from build123d import *

# Parameters (mm, degrees)
BOSS_EXTRUDE2_DEPTH = 87
CUT_EXTRUDE1_DEPTH  = 29.5
SKETCH3_R           = 1
CUT_EXTRUDE2_DEPTH  = 130.771336418
SKETCH4_R           = 1.7
CUT_EXTRUDE3_DEPTH  = 10
BOSS_EXTRUDE3_START = 2
BOSS_EXTRUDE3_DEPTH = 2
BOSS_EXTRUDE4_START = 6
BOSS_EXTRUDE4_DEPTH = 6
SKETCH7_W           = 73
SKETCH7_H           = 5.446782016
SKETCH7_H_2         = 6
CUT_EXTRUDE4_DEPTH  = 7
SKETCH8_R           = 1
CUT_EXTRUDE5_DEPTH  = 136.438914135
SKETCH9_R           = 2.5
CUT_EXTRUDE6_DEPTH  = 32
SKETCH11_W          = 10.498637593
SKETCH11_H          = 26.999999931
BOSS_EXTRUDE6_DEPTH = 23
SKETCH12_W          = 73
SKETCH12_H          = 6
SKETCH12_H_2        = 5.446782016
BOSS_EXTRUDE7_DEPTH = 14


with BuildPart() as part:
    # Sketch1 → Boss-Extrude2 (new body)
    with BuildSketch(Plane(origin=(89.94373008, 0, 0), x_dir=(0, 0, -1), z_dir=(1, 0, 0))):
        with BuildLine():
            Line((-104.016306216, 83.836001664), (-104.016306216, 0.836001664))
            ThreePointArc((-104.016306216, 0.836001664), (-62.516306216, 42.336001664), (-104.016306216, 83.836001664))
        make_face()
    extrude(amount=-BOSS_EXTRUDE2_DEPTH)

    # Sketch2 → Cut-Extrude1 (cut)
    with BuildSketch(Plane.XY.offset(104.016306216)):
        with BuildLine():
            Line((89.94373008, 55.836001595), (79.445092487, 55.836001664))
            Line((79.445092487, 55.836001664), (40.551337791, 64.805487997))
            ThreePointArc((40.551337791, 64.805487997), (5.067466824, 42.109927869), (40.551337791, 19.414367741))
            Line((40.551337791, 19.414367741), (79.445092487, 28.836001664))
            Line((79.445092487, 28.836001664), (89.94373008, 28.836001664))
            Line((89.94373008, 28.836001664), (89.94373008, 55.836001595))
        make_face()
    extrude(amount=-CUT_EXTRUDE1_DEPTH, mode=Mode.SUBTRACT)

    # Sketch3 → Cut-Extrude2 (cut, through all)
    with BuildSketch(Plane(origin=(0, 0, 62.516306216), x_dir=(-1, 0, 0), z_dir=(0, 0, -1))):
        with Locations(Location((-42.657418818, 50.264258545, 0), (0, 0, 90))):
            Circle(SKETCH3_R)
        with Locations(Location((-21.913136148, 54.699879864, 0), (0, 0, 90))):
            Circle(SKETCH3_R)
        with Locations(Location((-38.2217975, 29.519975875, 0), (0, 0, 90))):
            Circle(SKETCH3_R)
        with Locations(Location((-17.477514829, 33.955597193, 0), (0, 0, 90))):
            Circle(SKETCH3_R)
    extrude(amount=-CUT_EXTRUDE2_DEPTH, mode=Mode.SUBTRACT)

    # Sketch4 → Cut-Extrude3 (cut)
    with BuildSketch(Plane(origin=(0, 0, 62.516306216), x_dir=(-1, 0, 0), z_dir=(0, 0, -1))):
        with Locations(Location((-42.657418818, 50.264258545, 0), (0, 0, 90))):
            Circle(SKETCH4_R)
        with Locations(Location((-21.913136148, 54.699879864, 0), (0, 0, 90))):
            Circle(SKETCH4_R)
        with Locations(Location((-38.2217975, 29.519975875, 0), (0, 0, 90))):
            Circle(SKETCH4_R)
        with Locations(Location((-17.477514829, 33.955597193, 0), (0, 0, 90))):
            Circle(SKETCH4_R)
    extrude(amount=-CUT_EXTRUDE3_DEPTH, mode=Mode.SUBTRACT)

    # Sketch5 → Boss-Extrude3 (add)
    with BuildSketch(Plane(origin=(89.94373008, 0, 0), x_dir=(0, 0, -1), z_dir=(1, 0, 0)).offset(BOSS_EXTRUDE3_START)):
        with BuildLine():
            Line((-104.016306216, 55.836001595), (-104.016306216, 47.336001664))
            ThreePointArc((-104.016306216, 47.336001664), (-99.016306216, 42.336001664), (-104.016306216, 37.336001664))
            Line((-104.016306216, 37.336001664), (-104.016306216, 28.836001664))
            Line((-104.016306216, 28.836001664), (-104.016306216, 0.836001664))
            ThreePointArc((-104.016306216, 0.836001664), (-62.516306216, 42.336001664), (-104.016306216, 83.836001664))
            Line((-104.016306216, 83.836001664), (-104.016306216, 55.836001595))
        make_face()
    extrude(amount=-BOSS_EXTRUDE3_DEPTH)

    # Sketch6 → Boss-Extrude4 (add)
    with BuildSketch(Plane(origin=(91.94373008, 0, 0), x_dir=(0, 0, -1), z_dir=(1, 0, 0)).offset(BOSS_EXTRUDE4_START)):
        with BuildLine():
            Line((-104.016306216, 56.336001664), (-104.016306216, 47.336001664))
            ThreePointArc((-104.016306216, 47.336001664), (-99.016306216, 42.336001664), (-104.016306216, 37.336001664))
            Line((-104.016306216, 37.336001664), (-104.016306216, 28.336001664))
            ThreePointArc((-104.016306216, 28.336001664), (-90.016306216, 42.336001664), (-104.016306216, 56.336001664))
        make_face()
    extrude(amount=-BOSS_EXTRUDE4_DEPTH)

    # Sketch7 → Cut-Extrude4 (cut)
    with BuildSketch(Plane.XY.offset(104.016306216)):
        with Locations((47.44373008, 76.112610656)):
            Rectangle(SKETCH7_W, SKETCH7_H)
        with Locations((47.44373008, 8.836001664)):
            Rectangle(SKETCH7_W, SKETCH7_H_2)
    extrude(amount=-CUT_EXTRUDE4_DEPTH, mode=Mode.SUBTRACT)

    # Sketch8 → Cut-Extrude5 (cut, through all)
    with BuildSketch(Plane(origin=(0, 0, 62.516306216), x_dir=(-1, 0, 0), z_dir=(0, 0, -1))):
        with Locations(Location((-84.94373008, 65.836001664, 0), (0, 0, 90))):
            Circle(SKETCH8_R)
        with Locations(Location((-84.94373008, 17.836001664, 0), (0, 0, 90))):
            Circle(SKETCH8_R)
        with Locations(Location((-9.94373008, 65.836001664, 0), (0, 0, 90))):
            Circle(SKETCH8_R)
        with Locations(Location((-9.94373008, 17.836001664, 0), (0, 0, 90))):
            Circle(SKETCH8_R)
    extrude(amount=-CUT_EXTRUDE5_DEPTH, mode=Mode.SUBTRACT)

    # Sketch9 → Cut-Extrude6 (cut)
    with BuildSketch(Plane(origin=(0, 0, 62.516306216), x_dir=(-1, 0, 0), z_dir=(0, 0, -1))):
        with Locations(Location((-84.94373008, 65.836001664, 0), (0, 0, 90))):
            Circle(SKETCH9_R)
        with Locations(Location((-84.94373008, 17.836001664, 0), (0, 0, 90))):
            Circle(SKETCH9_R)
        with Locations(Location((-9.94373008, 65.836001664, 0), (0, 0, 90))):
            Circle(SKETCH9_R)
        with Locations(Location((-9.94373008, 17.836001664, 0), (0, 0, 90))):
            Circle(SKETCH9_R)
    extrude(amount=-CUT_EXTRUDE6_DEPTH, mode=Mode.SUBTRACT)

    # Sketch11 → Boss-Extrude6 (add)
    with BuildSketch(Plane.XY.offset(74.516306216)):
        with Locations((84.694411284, 42.33600163)):
            Rectangle(SKETCH11_W, SKETCH11_H)
    extrude(amount=BOSS_EXTRUDE6_DEPTH)

    # Sketch12 → Boss-Extrude7 (add)
    with BuildSketch(Plane(origin=(0, 0, 97.016306216), x_dir=(-1, 0, 0), z_dir=(0, 0, -1))):
        with Locations((-47.44373008, 8.836001664)):
            Rectangle(SKETCH12_W, SKETCH12_H)
        with Locations((-47.44373008, 76.112610656)):
            Rectangle(SKETCH12_W, SKETCH12_H_2)
    extrude(amount=-BOSS_EXTRUDE7_DEPTH)


solid = part.part
Design review of the part built by this model. Coordinates are the model's own, in mm. A direction names the side the tool comes from. Coordinates: 2 decimals unless noted, no trailing zeros. Write each loop counter-clockwise with the first axis right and the second up, starting at its lowest first coordinate (ties: lowest second). Pieces come first, ordered by that corner, then holes. Notation, with made-up numbers: (56.5, 5) - (87.5, 5) arc R7 ccw to (87.5, 15) - close; hole circle Ø2 at (46, 52). An arc over 180 degrees is marked (long way). Use one line per item in the form item = value.
Q1. Consider section B-B (z = 88.5). Write out the cut boundary in (x, y), plus the area to 3 significant figures.
Taken from the geometry:
outline = (2.94, 3.85) - (91.94, 3.85) - (91.94, 80.83) - (2.94, 80.83) - close; hole circle Ø5 at (9.94, 17.84); hole circle Ø5 at (9.94, 65.84); hole (40.55, 19.41) - (79.45, 28.84) - (79.45, 55.84) - (40.55, 64.81) arc R25 ccw (long way) to start; hole circle Ø5 at (84.94, 17.84); hole circle Ø5 at (84.94, 65.84)
area = 3,870 mm^2
Q2. Insertion check: pin 1 Ø2.5 at (x, y) = (42.66, 50.26) entering from -Z; pin 2 Ø8 at (x, y) = (9.94, 65.84) entering from +Z; pin 3 Ø4 at (x, y) = (9, 17) entering from -Z; pin 4 Ø1.7 at (x, y) = (17.5, 34) entering from -Z. Each pin has a flat end and moves straight along its axis. Give the tip position at first contact, or say it passes through.
Taken from the geometry:
pin_1 = 72.52
pin_2 = 104.02
pin_3 = 70.18
pin_4 = through
Q3. Consider section A-A (z = 107.5). Write out the cut boundary in (x, y), plus the area to 3 significant figures.
Taken from the geometry:
outline = (10.94, 5.84) - (83.94, 5.84) - (83.94, 11.84) - (10.94, 11.84) - close; (10.94, 73.39) - (83.94, 73.39) - (83.94, 78.84) - (10.94, 78.84) - close
area = 836 mm^2
Q4. Machinability: for faces 1 (the flat face through (48, 5.836, 107)), 2 (the flat face through (89.944, 42.5, 98.6)), 3 (the flat face through (10.944, 9, 107)), which of the approach directions +Z, -Z, +X, -X, +Y, -Y give a long, thin tool a straight path to every point of the face, cutting with its end or side? Answer none if there is none.
Taken from the geometry:
face_1 = +Z, +X, -X, -Y
face_2 = +Z
face_3 = +Z, -X, +Y, -Y
Q5. Consider section C-C (y = 10). Write out the cut boundary in (x, z).
Taken from the geometry:
outline = (2.94, 78) - (91.94, 78) - (91.94, 104.02) - (83.94, 104.02) - (83.94, 111.02) - (10.94, 111.02) - (10.94, 104.02) - (2.94, 104.02) - close
Q6. The part is to be moulded in two halves that separate along Y. For faces 4 (the flat face through (48, 76, 111.016)), 5 (the cylindrical face through (48.067, 41.423, 62.526)), 6 (the cylindrical face through (37.57, 31.09, 68.22)), say which applies: +Y half, -Y half, draft (parallel to the pull), parting line (faces both ways), or undercut.
Taken from the geometry:
face_4 = draft
face_5 = parting line
face_6 = undercut
Q7. For probe 1 along X at (y, z) = (19, 99.5); probe 2 along X at (y, z) = (39, 94); probe 3 along Z at (x, y) = (31, 35.5), list the stretches that pass through material, from the lowest coordinate up.
Taken from the geometry:
probe_1 = 2.94 to 20.53, 39.6 to 91.94
probe_2 = 2.94 to 5.26, 79.45 to 97.94
probe_3 = 63.08 to 74.52
